Autodesk Inventor part; units mm, degrees
ref_plane "YZ Plane" through (0, 0, 0) normal (1, 0, 0) x (0, 1, 0)
ref_plane "XZ Plane" through (0, 0, 0) normal (0, 1, 0) x (-1, 0, 0)
ref_plane "XY Plane" through (0, 0, 0) normal (0, 0, 1) x (1, 0, 0)
sketch "スケッチ1" plane through (0, 0, 0) normal (0, 0, 1) x (1, 0, 0)
  circle A0 centre (0, 0) radius 3
  dimension "d0" = 6
extrude "押し出し1" add sketch "スケッチ1" along normal blind 45
hole "穴1" at (0, 0, 0) direction (0, 0, 1) diameter 3 depth 6 tip angle 118
sketch "スケッチ2" plane through (0, 0, 45) normal (0, 0, 1) x (1, 0, 0)
  circle A0 centre (0, 0) radius 3
hole "穴2" at (0, 0, 45) direction (0, 0, -1) diameter 3 depth 6 tip angle 118
properties part number "スペーサ　m3-l45" material "アルミニウム 2014-T4"
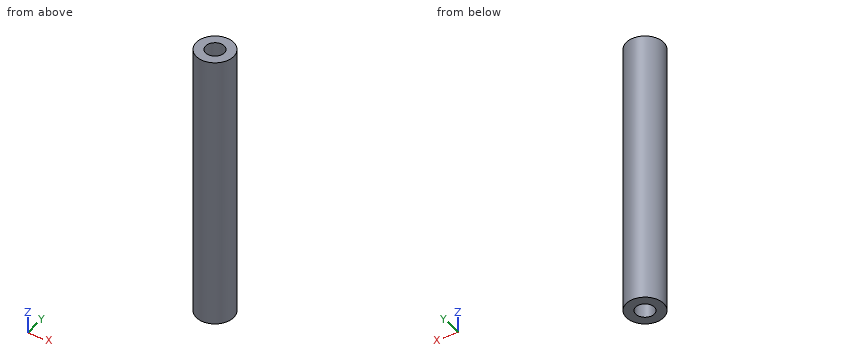
Source: CAD feature listing. Evaluate the final solid. Frame: model axes, mm. Coordinates: 2 decimals unless noted, no trailing zeros. Loops run counter-clockwise (first coordinate to the right, second up) from the corner with the lowest first, then second, coordinate; pieces in that order, holes last. Notation, with made-up numbers: M 6,15.25 L 15,15.25 A20 ccw 15,51.25 Z; hole C 4,71 d9. An arc over 180 degrees is marked long. Put each result on its own line as item: value. Start each with the question number.
1) Cut plane A-A on z = 19.5. Return the cut outline in (x, y).
2) Contact query for flat-ended pins moving along their axis: pin 1 Ø1 at (x, z) = (-0.5, 27.5) entering from -Y; pin 2 Ø2.5 at (x, y) = (0, 0) entering from +Z; pin 3 Ø2.5 at (x, y) = (0, 0) entering from -Z; pin 4 Ø1 at (y, z) = (1.5, 21) entering from -X. Output: stop coordinate, or through.
3) Ray query, L1, parallel to Y at x = 0, z = 2.5; L2, parallel to Y at x = 0.2, z = 32; L3, parallel to X at y = 0.1, z = 16. Return the intervals inside material, ascending. Write a range as from..to.
4) Cut plane B-B on y = 1.9. Return the cut outline in (x, z).
5) Cut plane C-C on y = -2.3. Return the cut outline in (x, z).
The answers:
1. outline: C 0,0 d6
2. pin 1: stops at y = -3
2. pin 2: stops at z = 38.85
2. pin 3: stops at z = 6.15
2. pin 4: stops at x = -2.83
3. L1: y = -3..-1.5, 1.5..3
3. L2: y = -2.99..2.99
3. L3: x = -3..3
4. outline: M -2.32,0 L 2.32,0 L 2.32,45 L -2.32,45 Z
5. outline: M -1.93,0 L 1.93,0 L 1.93,45 L -1.93,45 Z
